Geometry check sheet. Reference: the model listing, model coordinates, mm. A direction names the side the tool comes from. Round coordinates to 2 decimals unless told otherwise and drop trailing zeros. Order: outer loops, then holes, each group sorted by start corner. A loop starts at its lowest first (then second) coordinate and runs counter-clockwise, first axis right, second up. Notation, with made-up numbers: (19.25, 8.25) -> (39.25, 8.25) arc R20 cw to (39.25, 39.25) -> close; hole circle Ø9 at (75.25, 83.25). An arc over 180 degrees is marked (long way). Answer as a JSON object with one key per item and string values. Group by question number.
from build123d import *

# Parameters (mm, degrees)
SKETCH1_R                       = 3
BOSS_EXTRUDE1_DEPTH             = 10
CHAMFER1_SIZE                   = 5
FILLET1_R                       = 3
M3_TAPPED_HOLE3_D               = 2.5
M3_TAPPED_HOLE3_DEPTH           = 7.5
M3_TAPPED_HOLE3_TIP             = 0.751075774
M3_TAPPED_HOLE3_ON_FACE_2_D     = 2.5
M3_TAPPED_HOLE3_ON_FACE_2_DEPTH = 7.5
M3_TAPPED_HOLE3_ON_FACE_2_TIP   = 0.751075774


with BuildPart() as part:
    # Sketch1 → Boss-Extrude1 (new body)
    with BuildSketch(Plane(origin=(0, 0, 0), x_dir=(0, 0, -1), z_dir=(1, 0, 0))):
        Polygon((-16.5, 65.5), (-16.5, 56.5), (-10, 56.5), (-10, 4.5), (-16.5, 4.5), (-16.5, -4.5), (6.5, -4.5), (6.5, 4.5), (0, 4.5), (0, 56.5), (6.5, 56.5), (6.5, 65.5), align=None)
        with Locations((-10, 0)):
            Circle(SKETCH1_R, mode=Mode.SUBTRACT)
        with BuildLine():
            ThreePointArc((-8, 26.5), (-5, 29.5), (-2, 26.5))
            Line((-2, 26.5), (-2, 9.5))
            ThreePointArc((-2, 9.5), (-5, 6.5), (-8, 9.5))
            Line((-8, 9.5), (-8, 26.5))
        make_face(mode=Mode.SUBTRACT)
        Circle(SKETCH1_R, mode=Mode.SUBTRACT)
        with BuildLine():
            Line((-2, 51.5), (-2, 34.5))
            ThreePointArc((-2, 34.5), (-5, 31.5), (-8, 34.5))
            Line((-8, 34.5), (-8, 51.5))
            ThreePointArc((-8, 51.5), (-5, 54.5), (-2, 51.5))
        make_face(mode=Mode.SUBTRACT)
        with Locations((-10, 61)):
            Circle(SKETCH1_R, mode=Mode.SUBTRACT)
        with Locations((0, 61)):
            Circle(SKETCH1_R, mode=Mode.SUBTRACT)
    extrude(amount=BOSS_EXTRUDE1_DEPTH)

    # Chamfer1
    chamfer1_edges = [part.edges().sort_by_distance(p)[0] for p in [
        (5, 4.5, 10),
        (5, 56.5, 10),
        (5, 56.5, 0),
        (5, 4.5, 0),
    ]]
    chamfer(chamfer1_edges, length=CHAMFER1_SIZE)

    # Fillet1
    # the kernel refuses this fillet: 3 mm, written as the material it adds along each edge
    with BuildSketch(Plane(origin=(0, 51.5, 0), x_dir=(0, 0.7071067811865468, -0.7071067811865482), z_dir=(1, 0, 0)), Plane(origin=(0, 9.5, 0), x_dir=(0, 1, 0), z_dir=(1, 0, 0))) as fillet1_piece_1:
        with BuildLine():
            CenterArc((FILLET1_R * 0.414213562373, -FILLET1_R), FILLET1_R, 90, 45)
            Line((-FILLET1_R * 0.292893218813, -FILLET1_R * 0.292893218813), (0, 0))
            Line((0, 0), (FILLET1_R * 0.414213562373, 0))
        make_face()
    extrude(amount=10)
    with BuildSketch(Plane(origin=(0, 9.5, 10), x_dir=(0, 1, 0), z_dir=(1, 0, 0)), Plane(origin=(0, 51.5, 10), x_dir=(0, 0.7071067811865468, 0.7071067811865482), z_dir=(1, 0, 0))) as fillet1_piece_2:
        with BuildLine():
            CenterArc((FILLET1_R * 0.414213562373, FILLET1_R), FILLET1_R, 225, 45)
            Line((-FILLET1_R * 0.292893218813, FILLET1_R * 0.292893218813), (0, 0))
            Line((0, 0), (FILLET1_R * 0.414213562373, 0))
        make_face()
    extrude(amount=10)
    # the kernel refuses this fillet: 3 mm, written as the material it takes off along each edge
    with BuildSketch(Plane(origin=(-6.495190528, 56.5, 16.5), x_dir=(0, 1, 0), z_dir=(1, 0, 0))) as fillet1_2_piece_1:
        with BuildLine():
            CenterArc((2.598076211, -3), FILLET1_R, 90, 60)
            Line((0, -1.5), (0, 0))
            Line((0, 0), (2.598076211, 0))
        make_face()
    extrude(amount=22.990381057, mode=Mode.SUBTRACT)
    with BuildSketch(Plane(origin=(-7.5, 65.5, 16.5), x_dir=(0, 0, -1), z_dir=(1, 0, 0)), Plane(origin=(-7.5, 65.5, -6.5), x_dir=(0, -1, 0), z_dir=(1, 0, 0))) as fillet1_2_piece_2:
        with BuildLine():
            CenterArc((FILLET1_R, -FILLET1_R), FILLET1_R, 90, 90)
            Line((0, -FILLET1_R), (0, 0))
            Line((0, 0), (FILLET1_R, 0))
        make_face()
    extrude(amount=25, mode=Mode.SUBTRACT)
    with BuildSketch(Plane(origin=(-6.495190528, 56.5, -6.5), x_dir=(0, 0, 1), z_dir=(1, 0, 0))) as fillet1_2_piece_3:
        with BuildLine():
            CenterArc((3, -2.598076211), FILLET1_R, 120, 60)
            Line((0, -2.598076211), (0, 0))
            Line((0, 0), (1.5, 0))
        make_face()
    extrude(amount=22.990381057, mode=Mode.SUBTRACT)
    with BuildSketch(Plane(origin=(-6.495190528, 4.5, -6.5), x_dir=(0, 0, 1), z_dir=(1, 0, 0))) as fillet1_2_piece_4:
        with BuildLine():
            CenterArc((3, 2.598076211), FILLET1_R, 180, 60)
            Line((0, 2.598076211), (0, 0))
            Line((0, 0), (1.5, 0))
        make_face()
    extrude(amount=22.990381057, mode=Mode.SUBTRACT)
    with BuildSketch(Plane(origin=(-7.5, -4.5, -6.5), x_dir=(0, 1, 0), z_dir=(1, 0, 0)), Plane(origin=(-7.5, -4.5, 16.5), x_dir=(0, 0, -1), z_dir=(1, 0, 0))) as fillet1_2_piece_5:
        with BuildLine():
            CenterArc((FILLET1_R, FILLET1_R), FILLET1_R, 180, 90)
            Line((0, FILLET1_R), (0, 0))
            Line((0, 0), (FILLET1_R, 0))
        make_face()
    extrude(amount=25, mode=Mode.SUBTRACT)
    with BuildSketch(Plane(origin=(-6.495190528, 4.5, 16.5), x_dir=(0, -1, 0), z_dir=(1, 0, 0))) as fillet1_2_piece_6:
        with BuildLine():
            CenterArc((2.598076211, 3), FILLET1_R, 210, 60)
            Line((0, 1.5), (0, 0))
            Line((0, 0), (2.598076211, 0))
        make_face()
    extrude(amount=22.990381057, mode=Mode.SUBTRACT)

    # M3 Tapped Hole3
    with Locations(Plane(origin=(5, 65.5, 5), x_dir=(0, 0, 1), z_dir=(0, 1, 0))):
        with Locations((0, 0)):
            Hole(M3_TAPPED_HOLE3_D / 2, depth=M3_TAPPED_HOLE3_DEPTH)
            with Locations((0, 0, -(M3_TAPPED_HOLE3_DEPTH + M3_TAPPED_HOLE3_TIP / 2))):  # 118° drill point
                Cone(0, M3_TAPPED_HOLE3_D / 2, M3_TAPPED_HOLE3_TIP, mode=Mode.SUBTRACT)

    # M3 Tapped Hole3 on face 2
    with Locations(Plane(origin=(5, -4.5, 5), x_dir=(0, 0, -1), z_dir=(0, -1, 0))):
        with Locations((0, 0)):
            Hole(M3_TAPPED_HOLE3_ON_FACE_2_D / 2, depth=M3_TAPPED_HOLE3_ON_FACE_2_DEPTH)
            with Locations((0, 0, -(M3_TAPPED_HOLE3_ON_FACE_2_DEPTH + M3_TAPPED_HOLE3_ON_FACE_2_TIP / 2))):  # 118° drill point
                Cone(0, M3_TAPPED_HOLE3_ON_FACE_2_D / 2, M3_TAPPED_HOLE3_ON_FACE_2_TIP, mode=Mode.SUBTRACT)


solid = part.part
Item 1: Set-up check for faces 1 (the flat face through (5, 43, 8)), 2 (the flat face through (4.9, 6.5, 13)), 3 (the cylindrical face through (3.78, -0.7, 4.73)), 4 (the flat face through (4.9, 6.5, -3)): record each of +Z, -Z, +X, -X, +Y, -Y from which the full face is reachable in a straight line by a thin tool's end or side.
Item 2: Sectioned sample at C-C, the plane y = 16.5. Enter the section's corners in (x, z).
Item 3: Depth check by flat-ended pin: pin 1 Ø3.5 at (y, z) = (0, 10) entering from -X; pin 2 Ø3 at (x, y) = (5.5, 16.5) entering from +Z; pin 3 Ø4 at (x, y) = (1, 55.5) entering from +Z; pin 4 Ø2 at (x, z) = (5, 5) entering from +Y. Enter the tip coordinate at first touch or a pass-through.
Item 4: Sectioned sample at A-A, the plane y = 0. Enter the section's corners in (x, z).
Item 5: Thickness scan on L1, parallel to Z at x = 5, y = 61.25; L2, parallel to X at y = 63, z = 5; L3, parallel to Z at x = 9.25, y = 20.5. Record the ranges inside material, lowest first.
Item 6: Sectioned sample at D-D, the plane x = 1. Count the separate pieces of the cut face and the enclosed holes in it, then the cut area to 3 significant figures.
Item 7: Sectioned sample at B-B, the plane z = 9.25. Enter the section's corners in (x, y), then the cut area to 3 significant figures.
Item 8: Mould release check, pull along Y, two halves, no side actions. Record for faces 5 (the cylindrical face through (4.93, -3.6, 15.64)), 6 (the cylindrical face through (3.78, 61.7, 5.27)), 7 (the flat face through (4.9, 54.4, 12.9)): pulls with the +Y half, pulls with the -Y half, needs draft (parallel to the pull), parting line crosses it, or undercut.
Result:
{
 "1": {"face 1": "+X, -X", "face 2": "+Z, +X, -X", "face 3": "-Y", "face 4": "-Z, +X, -X"},
 "2": {"outline": "(0, 0) -> (10, 0) -> (10, 2) -> (0, 2) -> close; (0, 8) -> (10, 8) -> (10, 10) -> (0, 10) -> close"},
 "3": {"pin 1": "passes through", "pin 2": "stops at z = 10", "pin 3": "stops at z = 16.04", "pin 4": "stops at y = 57.85"},
 "4": {"outline": "(0, -6.5) -> (10, -6.5) -> (10, -3) -> (0, -3) -> close; (0, 3) -> (10, 3) -> (10, 7) -> (0, 7) -> close; (0, 13) -> (10, 13) -> (10, 16.5) -> (0, 16.5) -> close; hole circle Ø2.5 at (5, 5)"},
 "5": {"L1": "z = -6.5 to -2.99, 2.99 to 3.75, 6.25 to 7.01, 12.99 to 16.5", "L2": "x = 0 to 3.75, 6.25 to 10", "L3": "z = 0 to 2, 8 to 10"},
 "6": {"separate pieces": "1", "enclosed holes": "6", "area": "599 mm2"},
 "7": {"outline": "(0, -4.5) -> (10, -4.5) -> (10, -2.9) -> (0, -2.9) -> close; (0, 2.9) -> (10, 2.9) -> (10, 58.1) -> (0, 58.1) -> close; (0, 63.9) -> (10, 63.9) -> (10, 65.5) -> (0, 65.5) -> close", "area": "584 mm2"},
 "8": {"face 5": "pulls with the -Y half", "face 6": "needs draft", "face 7": "undercut"}
}
